Work out the finished part from the listing and answer in its coordinate system (mm). A direction names the side the tool comes from. Coordinates: 2 decimals unless noted, no trailing zeros. Order: outer loops, then holes, each group sorted by start corner. A loop starts at its lowest first (then second) coordinate and runs counter-clockwise, first axis right, second up. Notation, with made-up numbers: (56.25, -21) -> (69.25, -21) arc R22 ccw to (69.25, 2) -> close; hole circle Ø8 at (25.5, 37.5). An arc over 180 degrees is marked (long way). Use one line per item in the form item = value.
from build123d import *

# Parameters (mm, degrees)
F0_W     = 72
F0_H     = 35
F1_DEPTH = 26
F2_R     = 2.215241
F2_R_2   = 2.584448
F3_DEPTH = 25
F4_R     = 1
F5_DEPTH = 25


with BuildPart() as f1:
    # F0 (on Top) → F1 (new body)
    with BuildSketch(Plane.XY):
        Rectangle(F0_W, F0_H)
    extrude(amount=F1_DEPTH)

    # F2 (on face) → F3 (join)
    with BuildSketch(Plane.XZ.offset(17.5)):
        with Locations((32.055214, 22.994446)):
            Circle(F2_R)
        with Locations((31.794146, 3.67538)):
            Circle(F2_R_2)
    extrude(amount=F3_DEPTH)

    # F4 (on face) → F5 (join)
    with BuildSketch(Plane(origin=(0, 17.5, 0), x_dir=(-1, 0, 0), z_dir=(0, 1, 0))):
        with Locations((-33.889978, 24.676624)):
            Circle(F4_R)
        with Locations((-33.882375, 18.111377)):
            Circle(F4_R)
        with Locations((-33.944174, 13.035096)):
            Circle(F4_R)
        with Locations((-33.705986, 3.123124)):
            Circle(F4_R)
    extrude(amount=F5_DEPTH)


solid = f1.part
(1) Which of the six approach directions +Z, -Z, +X, -X, +Y, -Y give full straight-line access (tool end or side, diameter ignored) to faces 4 (the cylindrical face through (34.943, 29.825, 13.079)), 5 (the flat face through (36, 0, 13)), 6 (the cylindrical face through (30.297, -29.825, 21.647))?
Data:
face_4 = +Y
face_5 = +Z, -Z, +X, +Y, -Y
face_6 = -Y
(2) The mould has two halves that part along Z. Classify faces 1 (the cylindrical face through (32.75, 29.82, 3.42)), 2 (the flat face through (-1, 0, 0)), 3 (the flat face through (34, 42.5, 3)): released by +Z, released by -Z, zero draft, split by the parting line, or undercut.
Data:
face_1 = undercut
face_2 = released by -Z
face_3 = zero draft
(3) Straight lines are drawn through the part: line 1 along Y through (x, z) = (-3, 21.75); line 2 along Y through (x, z) = (30, 4.25); line 3 along X through (y, z) = (21.5, 17.25). For each, find the intervals that lie inside material, in ascending order.
Data:
line_1 = -17.5 to 17.5
line_2 = -42.5 to 17.5
line_3 = 33.37 to 34.39
(4) Section A-A on x = 27 is taken. Write down the section's boundary in (y, z).
Data:
outline = (-17.5, 0) -> (17.5, 0) -> (17.5, 26) -> (-17.5, 26) -> close
(5) Each of these flat-tipped pins is pushed along its axis until it touches: P1, Ø6, axis at x = -11.5, z = 19, coming from the +Y side; P2, Ø12, axis at x = 14.5, z = 23, coming from the -Y side. Where does it stop, or does it pass through?
Data:
P1 = 17.5
P2 = -17.5
(6) Section B-B on y = 34.5 is taken. Write down the section's boundary in (x, z).
Data:
outline = circle Ø2 at (33.71, 3.12); circle Ø2 at (33.88, 18.11); circle Ø2 at (33.89, 24.68); circle Ø2 at (33.94, 13.04)
